Autodesk Inventor part; units mm, degrees
ref_plane "Work Plane1" through (0, 20.2672, 186.8236) normal (0, 0, -1) x (-1, 0, 0)
ref_plane "YZ Plane" through (0, 0, 0) normal (1, 0, 0) x (0, 1, 0)
ref_plane "XZ Plane" through (0, 0, 0) normal (0, 1, 0) x (-1, 0, 0)
sketch "Sketch1" plane through (0, 0, 0) normal (1, 0, 0) x (0, 1, 0)
  line L0 (150.2672, 51.8236) -> (150.2672, 81.8236)
  line L1 (150.2672, 51.8236) -> (20.2672, 51.8236)
  line L2 (20.2672, 51.8236) -> (20.2672, 201.8236)
  line L3 (20.2672, 201.8236) -> (30.2672, 201.8236)
  line L4 (30.2672, 201.8236) -> (50.2672, 172.1724)
  line L5 (50.2672, 172.1724) -> (50.2672, 81.8236)
  line L6 (50.2672, 81.8236) -> (150.2672, 81.8236)
  dimension "d1" = 30
  dimension "d2" = 130
  dimension "d3" = 150
  dimension "d4" = 56
  dimension "d5" = 20
  dimension "d6" = 30
extrude "Extrusion1" add sketch "Sketch1" along normal blind 200
ref_plane "Work Plane1" through (0, 20.2672, 186.8236) normal (0, 0, -1) x (-1, 0, 0)
sketch "Sketch2" plane through (0, 50.2672, 172.1724) normal (0, 0.829, 0.5592) x (1, 0, 0)
  line L0 (200, -35.7658) -> (200, 0)
  circle A0 centre (150, -17.6726) radius 4
  circle A1 centre (50, -17.6726) radius 4
  line L1 (-20, -17.6726) -> (260, -17.6726)
  dimension "d10" = 8
  dimension "d11" = 50
  dimension "d12" = 100
extrude "Extrusion2" cut sketch "Sketch2" against normal up to next
sketch "Sketch3" plane through (0, 50.2672, 81.8236) normal (0, 0, 1) x (1, 0, 0)
  line L0 (200, 0) -> (200, 100)
  line L1 (0, 100) -> (200, 100)
  line L2 (0, 100) -> (0, 0)
  line L3 (85, 100) -> (115, 100)
  line L4 (115, 100) -> (115, 65.4079)
  line L5 (85, 65.4079) -> (85, 100)
  arc A0 (85, 65.4079) -> (115, 65.4079) centre (100, 65.4079) ccw
  dimension "d15" = 30
  dimension "d16" = 100
extrude "Extrusion3" cut sketch "Sketch3" against normal up to next
hole "Hole1" at (175, 80.2672, 81.8236) direction (0, 0, -1) diameter 6 depth 85 tip angle 118
hole "Hole2" at (175, 110.2672, 81.8236) direction (0, 0, -1) diameter 9 depth 30 tip angle 118 counterbore diameter 18 counterbore depth 11
hole "Hole3" at (25, 80.2672, 81.8236) direction (0, 0, -1) diameter 9 depth 30 tip angle 118 counterbore diameter 18 counterbore depth 11
hole "Hole4" at (25, 110.2672, 81.8236) direction (0, 0, -1) diameter 6 depth 30 tip angle 118
hole "Hole5" at (100, 50.2672, 127.1724) direction (0, -1, 0) diameter 8 depth 30 tip angle 118 counterbore diameter 20 counterbore depth 11
properties part number "bracket"
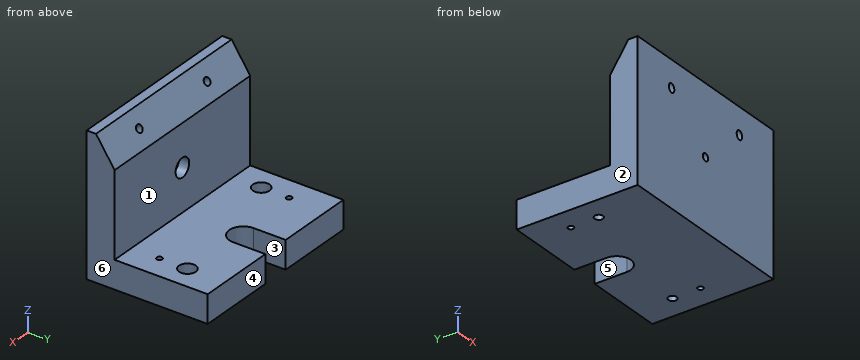
Part model, mm, in its own coordinate system. Face numbers are marked on the shaded views. A direction names the side the tool comes from. Coordinates: 2 decimals unless noted, no trailing zeros. Loops run counter-clockwise (first coordinate to the right, second up) from the corner with the lowest first, then second, coordinate; pieces in that order, holes last. Notation, with made-up numbers: (12, 26) - (59, 26) arc R19 ccw to (59, 51) - close; hole circle Ø8 at (13.5, -36). An arc over 180 degrees is marked (long way). Write each question's results on one line, items separated by ' | '. Start each with the question number.
Q1. Slice it at C-C on x = 175. Give the cut face in (y, z), and give its area (3 significant figures).
Q2. Slice it at A-A on y = 124.5. Give the cut face in (x, z), and give its area (3 significant figures).
Q3. Slice it at B-B on x = 100. Give the cut face in (y, z).
Q4. Probe line 1 along Y through (x, z) = (175, 57); line 2 along Y through (x, z) = (25, 58.5); line 3 along Z through (x, y) = (139.5, 81). List the from-to ranges inside material, lowest first.
Q5. Drop flat-ended pins along their axis: pin 1 Ø9 at (x, y) = (27.5, 83.5) entering from +Z; pin 2 Ø6 at (x, z) = (96.5, 125.5) entering from +Y; pin 3 Ø5 at (x, y) = (25, 110.27) entering from -Z; pin 4 Ø5 at (x, y) = (117, 111.5) entering from +Z. Give the stop position or say it passes through.
Q6. Which spindle directions (+Z, -Z, +X, -X, +Y, -Y) get a long thin tool onto all of the face, cutting with end or side? Do the marked faces 1, 2 and 3. Say none if no direction does.
Q7. Two-plate mould, pull along X, no slides. Class the marked faces 4, 5 and 6: +X half, -X half, draft (parallel to the pull), parting line (faces both ways), or undercut.
Q8. Slice it at D-D on x = 72. Give the cut face in (y, z).
Answer:
1) outline: (20.27, 51.82) - (77.27, 51.82) - (77.27, 81.82) - (50.27, 81.82) - (50.27, 172.17) - (30.27, 201.82) - (20.27, 201.82) - close; (83.27, 51.82) - (105.77, 51.82) - (105.77, 70.82) - (101.27, 70.82) - (101.27, 81.82) - (83.27, 81.82) - close; (114.77, 51.82) - (150.27, 51.82) - (150.27, 81.82) - (119.27, 81.82) - (119.27, 70.82) - (114.77, 70.82) - close | area: 6,650 mm2
2) outline: (0, 51.82) - (85, 51.82) - (85, 81.82) - (0, 81.82) - close; (115, 51.82) - (200, 51.82) - (200, 81.82) - (115, 81.82) - close | area: 5,100 mm2
3) outline: (20.27, 51.82) - (100.68, 51.82) - (100.68, 81.82) - (50.27, 81.82) - (50.27, 117.17) - (39.27, 117.17) - (39.27, 123.17) - (20.27, 123.17) - close; (20.27, 131.17) - (39.27, 131.17) - (39.27, 137.17) - (50.27, 137.17) - (50.27, 172.17) - (30.27, 201.82) - (20.27, 201.82) - close
4) line 1: y = 20.27 to 77.27, 83.27 to 105.77, 114.77 to 150.27 | line 2: y = 20.27 to 75.77, 84.77 to 107.27, 113.27 to 150.27 | line 3: z = 51.82 to 81.82
5) pin 1: stops at z = 70.82 | pin 2: stops at y = 39.27 | pin 3: passes through | pin 4: stops at z = 81.82
6) face 1: +Z, +X, -X, +Y | face 2: +Z, -Z, -X, +Y, -Y | face 3: +Z, -Z, +Y
7) face 4: draft | face 5: undercut | face 6: +X half
8) outline: (20.27, 51.82) - (150.27, 51.82) - (150.27, 81.82) - (50.27, 81.82) - (50.27, 172.17) - (30.27, 201.82) - (20.27, 201.82) - close
